Can you work these out from the model? Positions are in its coordinate system, mm. Face numbers are marked on the shaded views. A direction names the side the tool comes from. Coordinates: 2 decimals unless noted, no trailing zeros. Write each loop counter-clockwise with the first axis right and the second up, starting at its lowest first coordinate (ties: lowest second). Pieces come first, ordered by that corner, then holes. Notation, with made-up numbers: (75.25, -30.75) -> (116.25, -30.75) arc R27 cw to (116.25, -5.75) -> close; hole circle Ø8 at (-11, -20.5). An arc over 180 degrees is marked (long way). Answer as CSV lines item,"result". Start each with the question number.
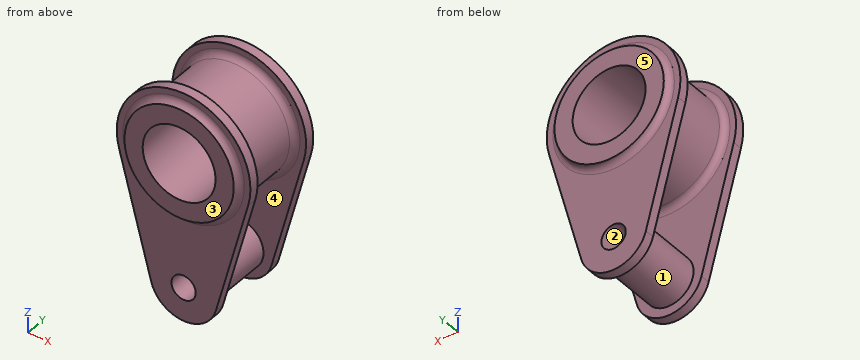
Autodesk Inventor part; units mm, degrees
ref_plane "YZ Plane" through (0, 0, 0) normal (1, 0, 0) x (0, 1, 0)
ref_plane "XZ Plane" through (0, 0, 0) normal (0, 1, 0) x (-1, 0, 0)
ref_plane "XY Plane" through (0, 0, 0) normal (0, 0, 1) x (1, 0, 0)
sketch "草图1" plane through (0, 0, 0) normal (0, 1, 0) x (-1, 0, 0)
  circle A0 centre (0, 0) radius 30
  circle A1 centre (0, 0) radius 45
  circle A2 centre (0, -106) radius 10
  circle A3 centre (0, 0) radius 55
  arc A4 (-26.5584, -113.1344) -> (26.5584, -113.1344) centre (0, -106) ccw
  line L0 (53.1168, -14.2689) -> (26.5584, -113.1344)
  line L1 (-53.1168, -14.2689) -> (-26.5584, -113.1344)
  circle A5 centre (0, -106) radius 20
  dimension "d0" = 60
  dimension "d1" = 90
  dimension "d3" = 20
  dimension "d4" = 110
  dimension "d5" = 55
  dimension "d8" = 40
extrude "拉伸2" add sketch "草图1" along normal blind 70 contours A5
extrude "拉伸3" add sketch "草图1" along normal blind 75 and the other way blind 5 contours A1
extrude "拉伸4" add sketch "草图1" along normal blind 8 contours A3 | A3 L0 A4 L1
sketch "草图2" plane through (0, 70, -106) normal (0, 1, 0) x (1, 0, 0)
  circle A0 centre (0, 0) radius 20
  circle A1 centre (0, 0) radius 10
  arc A2 (26.5584, 7.1344) -> (-26.5584, 7.1344) centre (0, 0) ccw
  arc A3 (-53.1168, -91.7311) -> (53.1168, -91.7311) centre (0, -106) ccw
  line L0 (53.1168, -91.7311) -> (26.5584, 7.1344)
  line L1 (26.5584, 7.1344) -> (53.1168, -91.7311)
  line L2 (-26.5584, 7.1344) -> (-53.1168, -91.7311)
  line L3 (-26.5584, 7.1344) -> (-53.1168, -91.7311)
  circle A4 centre (0, -106) radius 30
  circle A5 centre (0, 0) radius 10
  dimension "d19" = 60
extrude "拉伸5" add sketch "草图2" against normal blind 8 contours L0 A3 L2 A2
fillet "圆角1" radius 5 4 edges at (45, 70, 0) (45, 0, 0) (45, 62, 0) (45, 8, 0)
Q1. Which directions (+Z, -Z, +X, -X, +Y, -Y) give clear straight access to the entire face, cutting with the end or side of a thin tool? Please do the marked faces 1 and 2.
Q2. Imagine slicing it at C-C (y = 34). Write out the boundary of the cut face in (x, z), then the cut area to 3 significant figures.
Q3. For pin 1 (5 mm diameter, centred on x = -7, y = 12.5, fed in from +Z); pin 2 (8 mm diameter, centred on x = 36, y = 54.5, fed in from -Z); pin 3 (6 mm diameter, centred on y = 62, z = -105, fed in from +X); pin 4 (12 mm diameter, centred on x = 0, z = -106, fed in from -Y), each with a flat end and sliding along its axis, tell me the tip position at first contact or that it passes through.
Q4. If we mould it in two halves opening along Y, with no side actions, what happens to the marked faces 3, 4 and 5? For each: released by +Y, released by -Y, zero draft, split by the parting line, or undercut.
Q5. Imagine slicing it at D-D (x = 0). State how many separate pieces and enclosed holes the cut face has, then the cut area to 3 significant figures.
Q6. Imagine slicing it at B-B (y = 67). Write out the boundary of the cut face in (x, z).
Q7. I need wall thicknesses on L1, parallel to Z at x = 0, y = 22; L2, parallel to Y at x = 14.5, z = -56.5; L3, parallel to Z at x = 8.5, y = 50. Which ranges of each line are inside material? Lowest first, please.
Entries:
1,face 1,"none"
1,face 2,"+Y, -Y"
2,outline,"circle Ø90 at (0, 0); circle Ø40 at (0, -106); hole circle Ø60 at (0, 0); hole circle Ø20 at (0, -106)"
2,area,"4,480 mm2"
3,pin 1,"z = 45.5"
3,pin 2,"z = -31.64"
3,pin 3,"x = 29.55"
3,pin 4,"through"
4,face 3,"released by -Y"
4,face 4,"undercut"
4,face 5,"released by +Y"
5,separate pieces,"3"
5,enclosed holes,"1"
5,area,"4,780 mm2"
6,outline,"(-53.12, -14.27) -> (-26.56, -113.13) arc R27.5 ccw to (26.56, -113.13) -> (53.12, -14.27) arc R55 ccw (long way) to start; hole circle Ø60 at (0, 0); hole circle Ø20 at (0, -106)"
7,L1,"-126 to -116, -96 to -86, -45 to -30, 30 to 45"
7,L2,"0 to 8, 62 to 70"
7,L3,"-124.1 to -111.27, -100.73 to -87.9, -44.19 to -28.77, 28.77 to 44.19"
